```python
from build123d import *

# Parameters (mm, degrees)
CROQUIS1_R              = 9.5
CROQUIS1_R_2            = 1
SALIENTE_EXTRUIR1_DEPTH = 1.2
CROQUIS2_R              = 4.5
SALIENTE_EXTRUIR2_DEPTH = 2
SKETCH1_R               = 1.2
CUT_EXTRUDE2_DEPTH      = 5
CROQUIS3_R              = 3.35
CUT_EXTRUDE3_DEPTH      = 1.9


with BuildPart() as part:
    # Croquis1 → Saliente-Extruir1 (new body)
    with BuildSketch(Plane(origin=(0, 0, 0), x_dir=(1, 0, 0), z_dir=(0, 1, 0))):
        with Locations((-19.93721465, -8.386058239)):
            Circle(CROQUIS1_R)
        with Locations((-14.633913791, -3.08275738)):
            Circle(CROQUIS1_R_2, mode=Mode.SUBTRACT)
        with Locations((-14.633913791, -13.689359098)):
            Circle(CROQUIS1_R_2, mode=Mode.SUBTRACT)
        with Locations((-25.240515509, -13.689359098)):
            Circle(CROQUIS1_R_2, mode=Mode.SUBTRACT)
        with Locations((-25.240515509, -3.08275738)):
            Circle(CROQUIS1_R_2, mode=Mode.SUBTRACT)
    extrude(amount=SALIENTE_EXTRUIR1_DEPTH)

    # Croquis2 → Saliente-Extruir2 (add)
    with BuildSketch(Plane(origin=(0, 0, 0), x_dir=(-1, 0, 0), z_dir=(0, -1, 0))):
        with Locations((19.93721465, -8.386058239)):
            Circle(CROQUIS2_R)
    extrude(amount=SALIENTE_EXTRUIR2_DEPTH)

    # Sketch1 → Cut-Extrude2 (cut)
    with BuildSketch(Plane(origin=(0, 1.2, 0), x_dir=(1, 0, 0), z_dir=(0, 1, 0))):
        with Locations((-19.93721465, -8.386058239)):
            Circle(SKETCH1_R)
    extrude(amount=-CUT_EXTRUDE2_DEPTH, mode=Mode.SUBTRACT)

    # Croquis3 → Cut-Extrude3 (cut)
    with BuildSketch(Plane(origin=(0, -2, 0), x_dir=(-1, 0, 0), z_dir=(0, -1, 0))):
        with Locations((19.93721465, -8.386058239)):
            Circle(CROQUIS3_R)
    extrude(amount=-CUT_EXTRUDE3_DEPTH, mode=Mode.SUBTRACT)


solid = part.part
```
Build history of the part. All positions in model axes, mm. A direction names the side the tool comes from. Round coordinates to 2 decimals unless told otherwise and drop trailing zeros. Loops run counter-clockwise (first coordinate to the right, second up) from the corner with the lowest first, then second, coordinate; pieces in that order, holes last. Notation, with made-up numbers: M 12,-4 L 64,-4 A20 cw 64,25 Z; hole C 72,15 d3. An arc over 180 degrees is marked long. Answer as CSV lines item,"result".
1. 3-axis set-ups, long thin cutter, end or side, ignore diameter. For faces 1 (the cylindrical face through (-15.43, 0.59, 3.69)), 2 (the cylindrical face through (-16.59, -1.06, 8.24)): which of +Z, -Z, +X, -X, +Y, -Y reach the whole face in a straight line?
Resolved:
face 1,"+Y, -Y"
face 2,"-Y"
2. Flat gauge pins, fed straight in: P1, Ø2.5, axis at x = -25.24, z = 3.08, coming from the -Y side; P2, Ø4, axis at x = -19.94, z = 8.39, coming from the -Y side; P3, Ø1, axis at y = 0, z = 4, coming from the +X side. Where does each tip first touch, or does it go through?
Resolved:
P1,"stops at y = 0"
P2,"stops at y = -0.1"
P3,"stops at x = -11.27"
3. Cut at A-A on z = 9. Write the cut outline in (x, y), then the cut area to 3 significant figures.
Resolved:
outline,"M -29.42,0 L -24.4,0 L -24.4,-2 L -23.23,-2 L -23.23,-0.1 L -20.97,-0.1 L -20.97,1.2 L -29.42,1.2 Z; M -18.91,-0.1 L -16.64,-0.1 L -16.64,-2 L -15.48,-2 L -15.48,0 L -10.46,0 L -10.46,1.2 L -18.91,1.2 Z"
area,"25.4 mm²"
4. Wall check: probe 1 along Y at (x, z) = (-26.5, 11.75); probe 2 along Z at (x, y) = (-21, -0.9); probe 3 along X at (y, z) = (0.9, 8). Give the ranges that are in metal, low to high. Write a range as [from, to].
Resolved:
probe 1,"y = [0, 1.2]"
probe 2,"z = [4.01, 5.21], [11.56, 12.76]"
probe 3,"x = [-29.43, -21.07], [-18.8, -10.45]"
5. Cut at D-D on y = 0.3. Write the cut outline in (x, z), then the cut area to 3 significant figures.
Resolved:
outline,"C -19.94,8.39 d19; hole C -25.24,3.08 d2; hole C -25.24,13.69 d2; hole C -19.94,8.39 d2.4; hole C -14.63,3.08 d2; hole C -14.63,13.69 d2"
area,"266 mm²"
6. Cut at B-B on z = 14.25. Write the cut outline in (x, y).
Resolved:
outline,"M -27.41,0 L -26.07,0 L -26.07,1.2 L -27.41,1.2 Z; M -24.41,0 L -15.46,0 L -15.46,1.2 L -24.41,1.2 Z; M -13.81,0 L -12.46,0 L -12.46,1.2 L -13.81,1.2 Z"
7. Two-plate mould, pull along X, no slides. Class faces 3 (the cylindrical face through (-15.44, -0.99, 8.19)), 4 (the flat face through (-15.8, 0, 6.1)), 5 (the cylindrical face through (-15.37, 0.59, 13.01)): released by +X, released by -X, zero draft, split by the parting line, or undercut.
Resolved:
face 3,"split by the parting line"
face 4,"zero draft"
face 5,"undercut"
8. Cut at C-C on x = -16.25. Write the cut outline in (y, z).
Resolved:
outline,"M -2,5.81 L 0,5.81 L 0,-0.37 L 1.2,-0.37 L 1.2,17.14 L 0,17.14 L 0,10.97 L -2,10.97 Z"
